The model under review builds one solid part; all positions refer to its coordinate system, in mm. Give positions to 0.01 mm unless a question says otherwise; leave off trailing zeros. Order: outer loops, then holes, each group sorted by start corner. A loop starts at its lowest first (then second) coordinate and runs counter-clockwise, first axis right, second up. Notation, with made-up numbers: M 10.5,11 L 41.5,11 A30 ccw 41.5,36 Z; hole C -4,25.5 d6. An arc over 180 degrees is marked long. One line per question, with ' | ' between items. Start each with the question number.
1. Wall thickness on L1, parallel to X at y = 1.8, z = 0; L2, parallel to X at y = 3.1, z = 1: over which ranges is each line inside the solid? List them lowest first.
2. We need section B-B on x = 0. Write out the cut boundary in (y, z), then the cut area to 3 significant figures.
3. We need section C-C on x = -8. Write out the cut boundary in (y, z), then the cut area to 3 significant figures.
4. We need section D-D on y = 0.45. Write out the cut boundary in (x, z).
5. The part is to be moulded in two halves that separate along X. For faces 1 (the face through (3, 3.2, 0)), 2 (the face through (-1.45, 1.58, -0.06)), 3 (the face through (8.06, 1.58, -12.64)), say which applies: +X half, -X half, draft (parallel to the pull), parting line (faces both ways), or undercut.
6. We need section A-A on z = 0. Write out the cut boundary in (x, y).
7. Insertion check: P1, Ø1.5, axis at y = 1, z = 8, coming from the +X side; P2, Ø3, axis at x = 8, z = 0, coming from the -Y side. Each pin has a flat end and moves straight along its axis. Give the tip position at first contact, or say it passes through.
```python
from build123d import *

# Parameters (mm, degrees)
SKETCH1_R           = 14.99
SKETCH1_R_2         = 1.45
SKETCH1_R_3         = 1.2
BOSS_EXTRUDE1_DEPTH = 3.2


with BuildPart() as part:
    # Sketch1 → Boss-Extrude1 (new body)
    with BuildSketch(Plane(origin=(0, 0, 0), x_dir=(1, 0, 0), z_dir=(0, 1, 0))):
        Circle(SKETCH1_R)
        Circle(SKETCH1_R_2, mode=Mode.SUBTRACT)
        with Locations((0, 8)):
            Circle(SKETCH1_R_3, mode=Mode.SUBTRACT)
        with Locations((8, 0)):
            Circle(SKETCH1_R_3, mode=Mode.SUBTRACT)
        with Locations((0, -8)):
            Circle(SKETCH1_R_3, mode=Mode.SUBTRACT)
        with Locations((-8, 0)):
            Circle(SKETCH1_R_3, mode=Mode.SUBTRACT)
    extrude(amount=BOSS_EXTRUDE1_DEPTH)


solid = part.part
```
Entries:
1) L1: x = -14.99 to -9.2, -6.8 to -1.45, 1.45 to 6.8, 9.2 to 14.99 | L2: x = -14.96 to -8.66, -7.34 to -1.05, 1.05 to 7.34, 8.66 to 14.96
2) outline: M 0,-14.99 L 3.2,-14.99 L 3.2,-9.2 L 0,-9.2 Z; M 0,-6.8 L 3.2,-6.8 L 3.2,-1.45 L 0,-1.45 Z; M 0,1.45 L 3.2,1.45 L 3.2,6.8 L 0,6.8 Z; M 0,9.2 L 3.2,9.2 L 3.2,14.99 L 0,14.99 Z | area: 71.3 mm^2
3) outline: M 0,-12.68 L 3.2,-12.68 L 3.2,-1.2 L 0,-1.2 Z; M 0,1.2 L 3.2,1.2 L 3.2,12.68 L 0,12.68 Z | area: 73.5 mm^2
4) outline: C 0,0 d29.98; hole C -8,0 d2.4; hole C 0,0 d2.9; hole C 0,-8 d2.4; hole C 0,8 d2.4; hole C 8,0 d2.4
5) face 1: draft | face 2: undercut | face 3: parting line
6) outline: M -14.99,0 L -9.2,0 L -9.2,3.2 L -14.99,3.2 Z; M -6.8,0 L -1.45,0 L -1.45,3.2 L -6.8,3.2 Z; M 1.45,0 L 6.8,0 L 6.8,3.2 L 1.45,3.2 Z; M 9.2,0 L 14.99,0 L 14.99,3.2 L 9.2,3.2 Z
7) P1: stops at x = 13.12 | P2: stops at y = 0
